Check sheet for the modelled part. Datum: model origin and axes. Units: mm. A direction names the side the tool comes from. Round coordinates to 2 decimals unless told otherwise and drop trailing zeros. Answer in a Markdown table with one row per item.
Autodesk Inventor part; units mm, degrees
ref_plane "YZ Plane" through (0, 0, 0) normal (1, 0, 0) x (0, 1, 0)
ref_plane "XZ Plane" through (0, 0, 0) normal (0, 1, 0) x (-1, 0, 0)
ref_plane "XY Plane" through (0, 0, 0) normal (0, 0, 1) x (1, 0, 0)
sketch "스케치3" plane through (0, 0, 0) normal (0, 1, 0) x (-1, 0, 0)
  line L0 (35.7919, -14.8255) -> (14.8255, -35.7919)
  line L1 (14.8255, -35.7919) -> (-14.8255, -35.7919)
  line L2 (-14.8255, -35.7919) -> (-35.7919, -14.8255)
  line L3 (-35.7919, -14.8255) -> (-35.7919, 14.8255)
  line L4 (-35.7919, 14.8255) -> (-14.8255, 35.7919)
  line L5 (-14.8255, 35.7919) -> (14.8255, 35.7919)
  line L6 (14.8255, 35.7919) -> (35.7919, 14.8255)
  line L7 (35.7919, 14.8255) -> (35.7919, -14.8255)
  line L8 (32.5919, -13.5) -> (13.5, -32.5919)
  line L9 (13.5, -32.5919) -> (-13.5, -32.5919)
  line L10 (-13.5, -32.5919) -> (-32.5919, -13.5)
  line L11 (-32.5919, -13.5) -> (-32.5919, 13.5)
  line L12 (-32.5919, 13.5) -> (-13.5, 32.5919)
  line L13 (-13.5, 32.5919) -> (13.5, 32.5919)
  line L14 (13.5, 32.5919) -> (32.5919, 13.5)
  line L15 (32.5919, 13.5) -> (32.5919, -13.5)
  point P0 (0, 0)
  point P1 (0, 0)
  point P2 (0, 0)
  point P3 (0, 0)
  dimension "d43" = 27
  dimension "d44" = 3.2
extrude "돌출2" add sketch "스케치3" along normal blind 4.4 contours L0 L1 L2 L3 L4 L5 L6 L7 | L8 L9 L10 L11 L12 L13 L14 L15
sketch "스케치4" plane through (0, 4.4, 0) normal (0, 1, 0) x (1, 0, 0)
  line L0 (13.5, -32.5919) -> (-13.5, -32.5919)
  line L1 (-13.5, -32.5919) -> (-32.5919, -13.5)
  line L2 (-32.5919, -13.5) -> (-32.5919, 13.5)
  line L3 (-32.5919, 13.5) -> (-13.5, 32.5919)
  line L4 (-13.5, 32.5919) -> (13.5, 32.5919)
  line L5 (13.5, 32.5919) -> (32.5919, 13.5)
  line L6 (32.5919, 13.5) -> (32.5919, -13.5)
  line L7 (32.5919, -13.5) -> (13.5, -32.5919)
  line L8 (-14.1627, 34.1919) -> (14.1627, 34.1919)
  line L9 (14.1627, 34.1919) -> (34.1919, 14.1627)
  line L10 (34.1919, 14.1627) -> (34.1919, -14.1627)
  line L11 (34.1919, -14.1627) -> (14.1627, -34.1919)
  line L12 (14.1627, -34.1919) -> (-14.1627, -34.1919)
  line L13 (-14.1627, -34.1919) -> (-34.1919, -14.1627)
  line L14 (-34.1919, -14.1627) -> (-34.1919, 14.1627)
  line L15 (-34.1919, 14.1627) -> (-14.1627, 34.1919)
  line L16 (-13.3343, 32.1919) -> (13.3343, 32.1919)
  line L17 (13.3343, 32.1919) -> (32.1919, 13.3343)
  line L18 (32.1919, 13.3343) -> (32.1919, -13.3343)
  line L19 (32.1919, -13.3343) -> (13.3343, -32.1919)
  line L20 (13.3343, -32.1919) -> (-13.3343, -32.1919)
  line L21 (-13.3343, -32.1919) -> (-32.1919, -13.3343)
  line L22 (-32.1919, -13.3343) -> (-32.1919, 13.3343)
  line L23 (-32.1919, 13.3343) -> (-13.3343, 32.1919)
  line L24 (-35.7919, 14.8255) -> (-35.7919, -14.8255)
  point P0 (0, 0)
  point P1 (0, 0)
  point P2 (0, 0)
  point P3 (0, 0)
  dimension "d7" = 27
  dimension "d67" = 1.6
  dimension "d68" = 2
extrude "돌출3" cut sketch "스케치4" against normal blind 1.2 contours L0 L1 L2 L3 L4 L5 L6 L7 | L8 L9 L10 L11 L12 L13 L14 L15 | L16 L17 L18 L19 L20 L21 L22 L23
sketch "스케치5" plane through (0, 0, 0) normal (0, -1, 0) x (1, 0, 0)
  line L0 (10, 2.5) -> (20, 2.5)
  line L1 (20, 2.5) -> (20, -2.5)
  line L2 (20, -2.5) -> (10, -2.5)
  line L3 (10, -2.5) -> (10, 2.5)
  line L4 (10, 2.5) -> (20, -2.5) construction
  line L5 (20, 2.5) -> (10, -2.5) construction
  line L6 (-20, 2.5) -> (-10, 2.5)
  line L7 (-10, 2.5) -> (-10, -2.5)
  line L8 (-10, -2.5) -> (-20, -2.5)
  line L9 (-20, -2.5) -> (-20, 2.5)
  line L10 (-20, 2.5) -> (-10, -2.5) construction
  line L11 (-10, 2.5) -> (-20, -2.5) construction
  point P0 (0, 0)
  point P1 (15, 0)
  point P2 (-15, 0)
  dimension "d11" = 10
  dimension "d12" = 5
  dimension "d13" = 10
  dimension "d16" = 30
extrude "돌출4" add sketch "스케치5" along normal blind 10
sketch "스케치6" plane through (-10, 0, -2.5) normal (0, 0, -1) x (-1, 0, 0)
  circle A0 centre (5, -10) radius 5
  circle A1 centre (-25, -10) radius 5
  line L0 (-20, -10) -> (-30, -10)
  line L1 (10, -10) -> (0, -10)
  point P0 (-10, 0)
  dimension "d23" = 10
  dimension "d24" = 10
extrude "돌출5" add sketch "스케치6" against normal blind 5
sketch "스케치7" plane through (-10, 0, -2.5) normal (0, 0, -1) x (-1, 0, 0)
  circle A0 centre (5, -10) radius 1.25
  line L0 (10, 0) -> (10, -10)
  line L1 (0, 0) -> (10, 0)
  line L2 (4.7788, 0) -> (0, 0)
  circle A1 centre (-25, -10) radius 1.25
  point P0 (-10, 0)
  dimension "d27" = 2.5
  dimension "d28" = 5
  dimension "d31" = 30
extrude "돌출6" cut sketch "스케치7" against normal blind 5
sketch "스케치8" plane through (0, 0, 0) normal (0, -1, 0) x (1, 0, 0)
  circle A0 centre (0, -25) radius 1.25
  line L0 (-10, 2.5) -> (-10, -2.5)
  point P0 (0, 0)
  point P1 (-10, 0)
  dimension "d38" = 2.5
  dimension "d39" = 25
sketch "스케치9" plane through (0, 3.2, 0) normal (0, 1, 0) x (1, 0, 0)
  line L0 (-13.3343, 32.1919) -> (13.3343, 32.1919)
  line L1 (13.3343, 32.1919) -> (32.1919, 13.3343)
  line L2 (32.1919, 13.3343) -> (32.1919, -13.3343)
  line L3 (32.1919, -13.3343) -> (13.3343, -32.1919)
  line L4 (13.3343, -32.1919) -> (-13.3343, -32.1919)
  line L5 (-13.3343, -32.1919) -> (-32.1919, -13.3343)
  line L6 (-32.1919, -13.3343) -> (-32.1919, 13.3343)
  line L7 (-32.1919, 13.3343) -> (-13.3343, 32.1919)
  line L8 (-14.1627, 34.1919) -> (14.1627, 34.1919)
  line L9 (-12.0917, 29.1919) -> (12.0917, 29.1919)
  line L10 (12.0917, 29.1919) -> (29.1919, 12.0917)
  line L11 (29.1919, 12.0917) -> (29.1919, -12.0917)
  line L12 (29.1919, -12.0917) -> (12.0917, -29.1919)
  line L13 (12.0917, -29.1919) -> (-12.0917, -29.1919)
  line L14 (-12.0917, -29.1919) -> (-29.1919, -12.0917)
  line L15 (-29.1919, -12.0917) -> (-29.1919, 12.0917)
  line L16 (-29.1919, 12.0917) -> (-12.0917, 29.1919)
  point P0 (0, 0)
  point P1 (0, 0)
  point P2 (0, 0)
  dimension "d46" = 2
  dimension "d47" = 3
extrude "돌출8" add sketch "스케치9" along normal blind 0.6 contours L0 L1 L2 L3 L4 L5 L6 L7 | L9 L10 L11 L12 L13 L14 L15 L16
fillet "모깎기1" radius 1.2 16 edges at (-35.7919, 4.4, 0) (-25.3087, 4.4, 25.3087) (0, 4.4, 35.7919) (25.3087, 4.4, 25.3087) (35.7919, 4.4, 0) (25.3087, 4.4, -25.3087) (0, 4.4, -35.7919) (-25.3087, 4.4, -25.3087) (25.3087, 0, 25.3087) (0, 0, 35.7919) (-25.3087, 0, 25.3087) (-35.7919, 0, 0) (-25.3087, 0, -25.3087) (0, 0, -35.7919) (25.3087, 0, -25.3087) (35.7919, 0, 0)
sketch "스케치10" plane through (0, 0, 0) normal (0, -1, 0) x (1, 0, 0)
  line L0 (-20, 2.5) -> (-10, 2.5)
  line L1 (-10, -2.5) -> (-20, -2.5)
  line L2 (-20, 2.5) -> (-19, 2.5)
  line L3 (-19, 2.5) -> (-19, -2.5)
  line L4 (-19, -2.5) -> (-20, -2.5)
  line L5 (-20, -2.5) -> (-20, 2.5)
  line L6 (20, -2.5) -> (10, -2.5)
  line L7 (10, 2.5) -> (20, 2.5)
  line L8 (20, -2.5) -> (19, -2.5)
  line L9 (19, -2.5) -> (19, 2.5)
  line L10 (19, 2.5) -> (20, 2.5)
  line L11 (20, 2.5) -> (20, -2.5)
  point P0 (0, 0)
  dimension "d54" = 1
  dimension "d55" = 1
extrude "돌출9" cut sketch "스케치10" along normal blind 15
extrude "돌출10" cut sketch "스케치8" against normal blind 5
sketch "스케치11" plane through (0, 3.8, 0) normal (0, 1, 0) x (1, 0, 0)
  line L0 (-6.575, 15.8735) -> (6.575, 15.8735)
  line L1 (6.575, 15.8735) -> (15.8735, 6.575)
  line L2 (15.8735, 6.575) -> (15.8735, -6.575)
  line L3 (15.8735, -6.575) -> (6.575, -15.8735)
  line L4 (6.575, -15.8735) -> (-6.575, -15.8735)
  line L5 (-6.575, -15.8735) -> (-15.8735, -6.575)
  line L6 (-15.8735, -6.575) -> (-15.8735, 6.575)
  line L7 (-15.8735, 6.575) -> (-6.575, 15.8735)
  line L8 (-7.4034, 17.8735) -> (7.4034, 17.8735)
  line L9 (7.4034, 17.8735) -> (17.8735, 7.4034)
  line L10 (17.8735, 7.4034) -> (17.8735, -7.4034)
  line L11 (17.8735, -7.4034) -> (7.4034, -17.8735)
  line L12 (7.4034, -17.8735) -> (-7.4034, -17.8735)
  line L13 (-7.4034, -17.8735) -> (-17.8735, -7.4034)
  line L14 (-17.8735, -7.4034) -> (-17.8735, 7.4034)
  line L15 (-17.8735, 7.4034) -> (-7.4034, 17.8735)
  point P0 (0, 0)
  point P1 (0, 0)
  point P2 (0, 0)
  point P3 (0, 17.8735)
  dimension "d60" = 13.15
  dimension "d61" = 2
extrude "돌출11" cut sketch "스케치11" against normal blind 0.6
sketch "스케치12" plane through (0, 3.8, 0) normal (0, 1, 0) x (1, 0, 0)
  circle A0 centre (0, 0) radius 4
  dimension "d64" = 8
extrude "돌출12" cut sketch "스케치12" against normal up to surface (3.8 mm away)
equation "\"d55\" = d54"
properties part number "OV-PAM_top_2"
Item 1: Cross-section at A-A (x = 0). State how many separate pieces and enclosed holes the cut face has, and give its area (3 significant figures).
Result sheet:
| item | result |
|---|---|
| separate pieces | 3 |
| enclosed holes | 0 |
| area | 228 mm^2 |
Item 2: Set-up check for faces 1 (the flat face through (22.631, 3.496, -22.895)), 2 (the flat face through (19, -6, 0)), 3 (the flat face through (14, -7, 2.5)): record each of +Z, -Z, +X, -X, +Y, -Y from which the full face is reachable in a straight line by a thin tool's end or side.
Result sheet:
| item | result |
|---|---|
| face 1 | +Y |
| face 2 | +Z, -Z, +X, -Y |
| face 3 | +Z, +X, -X, -Y |
Item 3: Mould release check, pull along Z, two halves, no side actions. Record for faces 4 (the flat face through (0, 2, -35.792)), 5 (the flat face through (24.318, 3.808, 24.037)), 6 (the cylindrical face through (-25.2, 0.342, 24.907)): pulls with the +Z half, pulls with the -Z half, needs draft (parallel to the pull), parting line crosses it, or undercut.
Result sheet:
| item | result |
|---|---|
| face 4 | pulls with the -Z half |
| face 5 | undercut |
| face 6 | pulls with the +Z half |
Item 4: Scan lines: line 1 (Z direction, x = 0, y = 3.05); line 2 (Y direction, x = -15, z = -0.3); line 3 (X direction, y = 2.9, z = 0). Record each from-to range of solid material in increasing order. Write a range as [from, to].
Result sheet:
| item | result |
|---|---|
| line 1 | z = [-35.79, -26.25], [-23.75, -4], [4, 35.79] |
| line 2 | y = [-15, -11.25], [-8.75, 3.8] |
| line 3 | x = [-35.79, -4], [4, 35.79] |
Item 5: Depth check by flat-ended pin: P1, Ø4, axis at x = -9, y = -9.5, coming from the +Z side; P2, Ø4, axis at y = -3.5, z = -9.5, coming from the +X side; P3, Ø10, axis at x = -26.5, y = -4, coming from the -Z side; P4, Ø1.5, axis at y = -4.5, z = 0, coming from the +X side. Enter the tip coordinate at first touch or a pass-through.
Result sheet:
| item | result |
|---|---|
| P1 | stops at z = 2.5 |
| P2 | passes through |
| P3 | stops at z = -26.09 |
| P4 | stops at x = 19 |
